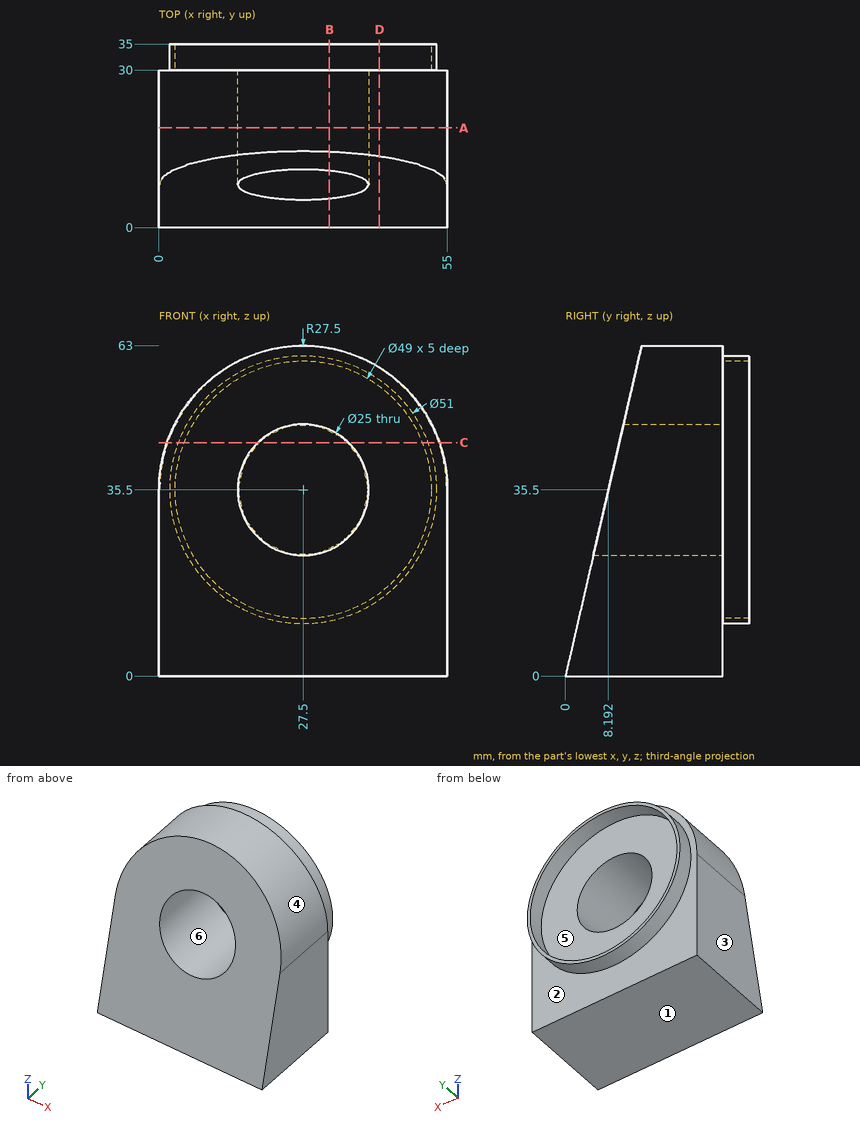
Part print with two shaded views. Sizes in mm from the minimum x, y, z corner. A direction names the side the tool comes from. Give positions to 0.01 mm unless a question says otherwise; leave off trailing zeros. Loops run counter-clockwise (first coordinate to the right, second up) from the corner with the lowest first, then second, coordinate; pieces in that order, holes last. Notation, with made-up numbers: (-34.5, 80.5) - (-3.5, 80.5) arc R10 ccw to (-3.5, 97.5) - close; hole circle Ø5 at (76.25, 80). An arc over 180 degrees is marked (long way). Put each result on its own line as item: value.
Q1. Slice it at D-D (x = 42). Give the cut face in (y, z) (1 decimal).
Filled in:
outline: (0, 0) - (30, 0) - (30, 14.5) - (35, 14.5) - (35, 15.8) - (30, 15.8) - (30, 55.2) - (35, 55.2) - (35, 56.5) - (30, 56.5) - (30, 58.9) - (13.6, 58.9) - close
Q2. Probe line 1 along Z through (x, y) = (27, 31) (1 decimal); line 2 along X through (y, z) = (31, 35) (1 decimal); line 3 along Z through (x, y) = (27, 18) (1 decimal). List the from-to ranges inside material, lowest first.
Filled in:
line 1: z = 10 to 11, 60 to 61
line 2: x = 2 to 3, 52 to 53
line 3: z = 0 to 23, 48 to 63
Q3. Slice it at A-A (y = 19). Give the cut face in (x, z).
Filled in:
outline: (0, 0) - (55, 0) - (55, 35.5) arc R27.5 ccw to (0, 35.5) - close; hole circle Ø25 at (27.5, 35.5)
Q4. Mould opens along Z. For the marked faces 3, 4, 5 and 6 say: pulls with the +Z half, pulls with the -Z half, needs draft (parallel to the pull), parting line crosses it, or undercut.
Filled in:
face 3: needs draft
face 4: pulls with the +Z half
face 5: undercut
face 6: undercut
Q5. Slice it at B-B (x = 32.5). Give the cut face in (y, z) (1 decimal).
Filled in:
outline: (0, 0) - (30, 0) - (30, 10.5) - (35, 10.5) - (35, 11.5) - (30, 11.5) - (30, 24) - (5.5, 24) - close; (10.8, 47) - (30, 47) - (30, 59.5) - (35, 59.5) - (35, 60.5) - (30, 60.5) - (30, 62.5) - (14.4, 62.5) - close
Q6. Tool access for the marked faces 1 and 2: list every direction of +Z, -Z, +X, -X, +Y, -Y with a clear straight run to the whole face (end or side of a thin tool).
Filled in:
face 1: -Z, +X, -X, +Y, -Y
face 2: +Y
Q7. Flat gauge pins, fed straight in: pin 1 (10 mm diameter, centred on y = 23, z = 48.5, fed in from -X); pin 2 (5 mm diameter, centred on x = 6, z = 15, fed in from -Y) (1 decimal); pin 3 (22.5 mm diameter, centred on x = 27.5, z = 35.5, fed in from +Y); pin 4 (3 mm diameter, centred on x = 44.5, z = 27.5, fed in from +Y). Where does each tip first touch, or does it go through?
Filled in:
pin 1: stops at x = 1.19
pin 2: stops at y = 2.9
pin 3: passes through
pin 4: stops at y = 30
Q8. Slice it at C-C (z = 44.5). Give the cut face in (x, y) (1 decimal), plus the area to 3 significant figures.
Filled in:
outline: (1.5, 10.3) - (18.8, 10.3) - (18.8, 30) - (4.7, 30) - (4.7, 35) - (3.6, 35) - (3.6, 30) - (1.5, 30) - close; (36.2, 10.3) - (53.5, 10.3) - (53.5, 30) - (51.4, 30) - (51.4, 35) - (50.3, 35) - (50.3, 30) - (36.2, 30) - close
area: 694 mm²
